The model under review builds one solid part; all positions refer to its coordinate system, in mm. Face numbers are marked on the shaded views. A direction names the side the tool comes from. Give positions to 0.01 mm unless a question says otherwise; leave off trailing zeros. Loops run counter-clockwise (first coordinate to the right, second up) from the corner with the lowest first, then second, coordinate; pieces in that order, holes last. Notation, with made-up numbers: M -27,22 L 26,22 A12 cw 26,39 Z; hole C -27.5,14.5 d5. An arc over 180 degrees is marked long. Return JSON: item names as keys, results as strings.
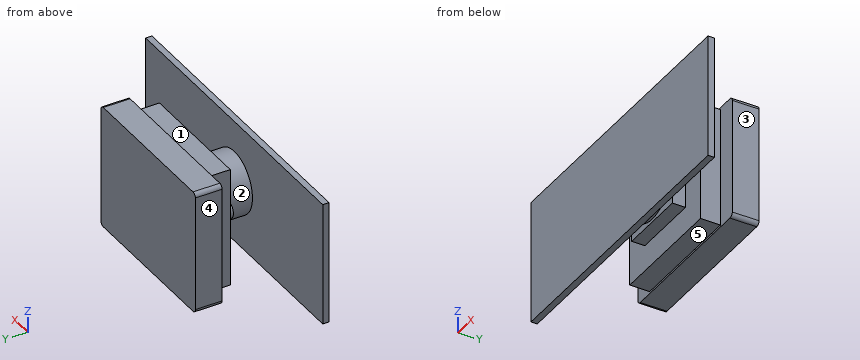
```python
from build123d import *

# Parameters (mm, degrees)
F0_W      = 40
F0_H      = 31
F1_DEPTH  = 6.7
F2_R      = 1
F3_W      = 30
F3_H      = 30
F4_DEPTH  = 5
F6_DEPTH  = 8.3
F7_R      = 7.725
F8_DEPTH  = 8.15
F9_W      = 75
F9_H      = 31
F10_DEPTH = 1.5748


with BuildPart() as f1:
    # F0 (on Front) → F1 (new body)
    with BuildSketch(Plane.XZ):
        Rectangle(F0_W, F0_H)
    extrude(amount=-F1_DEPTH)

    # F2
    f2_edges = [f1.edges().sort_by_distance(p)[0] for p in [
        (-20, 3.35, 15.5),
        (-20, 3.35, -15.5),
        (20, 3.35, 15.5),
        (20, 3.35, -15.5),
    ]]
    fillet(f2_edges, radius=F2_R)

    # F3 (on face) → F4 (join)
    with BuildSketch(Plane.XZ):
        Rectangle(F3_W, F3_H)
    extrude(amount=F4_DEPTH)

    # F5 (on face) → F6 (join)
    with BuildSketch(Plane.XZ):
        Polygon((8.625, 2.15), (8.625, 8.45), (-8.625, 8.45), (-8.625, 2.15), (-8.625, -2.15), (-8.625, -8.45), (8.625, -8.45), (8.625, -2.15), align=None)
        with BuildLine():
            ThreePointArc((8.625, -2.15), (10.775, 0), (8.625, 2.15))
            Line((8.625, 2.15), (8.625, -2.15))
        make_face()
        with BuildLine():
            Line((-8.625, -2.15), (-8.625, 2.15))
            ThreePointArc((-8.625, 2.15), (-10.775, 0), (-8.625, -2.15))
        make_face()
    extrude(amount=F6_DEPTH)

    # F7 (on face) → F8 (join)
    with BuildSketch(Plane.XZ.offset(8.3)):
        Circle(F7_R)
    extrude(amount=F8_DEPTH)

    # F9 (on face) → F10 (join)
    with BuildSketch(Plane.XZ.offset(16.45)):
        Rectangle(F9_W, F9_H)
    extrude(amount=-F10_DEPTH)


solid = f1.part
```
1) Tool access review of the marked faces 1, 2, 3, 4 and 5: name each direction out of +Z, -Z, +X, -X, +Y, -Y from which nothing blocks a thin tool from reaching the whole face with its end or side.
From the geometry:
{"face 1": "+Z, +X, -X", "face 2": "none", "face 3": "+Z, -Z, +X, +Y", "face 4": "+Z, -Z, -X, +Y", "face 5": "-Z, +X, -X"}
2) Consider section B-B on z = 12. Write out the cut boundary in (x, y), then the cut area to 3 significant figures.
From the geometry:
{"outline": "M -37.5,-16.45 L 37.5,-16.45 L 37.5,-14.88 L -37.5,-14.88 Z; M -20,0 L -15,0 L -15,-5 L 15,-5 L 15,0 L 20,0 L 20,6.7 L -20,6.7 Z", "area": "536 mm²"}
3) Wall thickness on L1, parallel to Y at x = 9, z = 7.5; L2, parallel to X at y = -1.25, z = -5.5; L3, parallel to Y at x = -18, z = 5.5: over which ranges is each line inside the solid? List them lowest first. Write a range as from..to.
From the geometry:
{"L1": "-16.45..-14.88, -5..6.7", "L2": "-15..15", "L3": "-16.45..-14.88, 0..6.7"}
4) Consider section D-D on z = 0. Write out the cut boundary in (x, y) (3 decimals), then the cut area to 3 significant figures.
From the geometry:
{"outline": "M -37.5,-16.45 L 37.5,-16.45 L 37.5,-14.875 L 7.725,-14.875 L 7.725,-8.3 L 10.775,-8.3 L 10.775,-5 L 15,-5 L 15,0 L 20,0 L 20,6.7 L -20,6.7 L -20,0 L -15,0 L -15,-5 L -10.775,-5 L -10.775,-8.3 L -7.725,-8.3 L -7.725,-14.875 L -37.5,-14.875 Z", "area": "709 mm²"}
5) Consider section C-C on y = 3.5. Write out the cut boundary in (x, z).
From the geometry:
{"outline": "M -20,-14.5 A1 ccw -19,-15.5 L 19,-15.5 A1 ccw 20,-14.5 L 20,14.5 A1 ccw 19,15.5 L -19,15.5 A1 ccw -20,14.5 Z"}
6) Insertion check: pin 1 (3.5 mm diameter, centred on y = -6.5, z = 4.5, fed in from -X); pin 2 (1.7 mm diameter, centred on x = 3, y = -6.5, fed in from +Z); pin 3 (3.5 mm diameter, centred on x = -0.5, y = -6, fed in from -Z). Each pin has a flat end and moves straight along its axis. Give the tip position at first contact, or say it passes through.
From the geometry:
{"pin 1": "x = -15", "pin 2": "z = 8.45", "pin 3": "z = -15"}
7) Consider section A-A on x = 13.5. Write out the cut boundary in (y, z).
From the geometry:
{"outline": "M -16.45,-15.5 L -14.88,-15.5 L -14.88,15.5 L -16.45,15.5 Z; M -5,-15 L 0,-15 L 0,-15.5 L 6.7,-15.5 L 6.7,15.5 L 0,15.5 L 0,15 L -5,15 Z"}
